from build123d import *

# Parameters (mm, degrees)
BOSS_EXTRUDE2_DEPTH     = 24
BOSS_EXTRUDE3_DEPTH     = 19
CUT_EXTRUDE1_DEPTH      = 1
BOSS_EXTRUDE4_DEPTH     = 50
SKETCH5_R               = 4
CUT_EXTRUDE2_DEPTH      = 55
SKETCH6_R               = 5
CUT_EXTRUDE3_DEPTH      = 25
CUT_EXTRUDE3_DEPTH_BACK = 25


with BuildPart() as part:
    # Sketch1 → Boss-Extrude2 (new body, symmetric)
    with BuildSketch(Plane.XY):
        Polygon((0, 0), (84, 0), (84, 19), (53, 19), (51.5, 16), (50, 19), (0, 19), align=None)
    extrude(amount=BOSS_EXTRUDE2_DEPTH, both=True)

    # Sketch2 → Boss-Extrude3 (add)
    with BuildSketch(Plane(origin=(0, 0, 0), x_dir=(1, 0, 0), z_dir=(0, 1, 0))):
        Polygon((84, 2), (89, 2), (100, 13.5), (100, 16.5), (89, 16.5), (89, 13.5), (84, 13.5), align=None)
    boss_extrude3 = extrude(amount=BOSS_EXTRUDE3_DEPTH)

    # Mirror1: Boss-Extrude3 across plane
    add(boss_extrude3.mirror(Plane.XY))

    # Sketch3 → Cut-Extrude1 (cut)
    with BuildSketch(Plane(origin=(0, 19, 0), x_dir=(1, 0, 0), z_dir=(0, 1, 0))):
        with BuildLine():
            Line((66, 12.5), (66, -12.5))
            ThreePointArc((66, -12.5), (63, -15.5), (60, -12.5))
            Line((60, -12.5), (60, 12.5))
            ThreePointArc((60, 12.5), (63, 15.5), (66, 12.5))
        make_face()
    extrude(amount=-CUT_EXTRUDE1_DEPTH, mode=Mode.SUBTRACT)

    # Sketch4 → Boss-Extrude4 (add)
    with BuildSketch(Plane(origin=(0, 0, 0), x_dir=(0, 0, -1), z_dir=(1, 0, 0))):
        Polygon((-18, 19), (-18, 32), (-24, 32), (-24, 38), (-13.5, 38), (-13.5, 43), (-16.5, 43), (-16.5, 54), (-13.5, 54), (-3.604820816, 41), (-3.604820816, 38), (0, 38), (0, 19), align=None)
    boss_extrude4 = extrude(amount=BOSS_EXTRUDE4_DEPTH)

    # Mirror2: Boss-Extrude4 across plane
    add(boss_extrude4.mirror(Plane.XY))

    # Sketch5 → Cut-Extrude2 (cut, through all)
    with BuildSketch(Plane(origin=(0, 0, 0), x_dir=(1, 0, 0), z_dir=(0, 1, 0))):
        with Locations((25, 0)):
            Circle(SKETCH5_R)
    extrude(amount=CUT_EXTRUDE2_DEPTH, mode=Mode.SUBTRACT)

    # Sketch6 → Cut-Extrude3 (cut, two sides)
    with BuildSketch(Plane.XY) as cut_extrude3_sk:
        with Locations((25, 25)):
            Circle(SKETCH6_R)
    extrude(amount=CUT_EXTRUDE3_DEPTH, mode=Mode.SUBTRACT)
    extrude(cut_extrude3_sk.sketch, amount=-CUT_EXTRUDE3_DEPTH_BACK, mode=Mode.SUBTRACT)


solid = part.part
For this review, take the finished solid that the model builds, in its own axes (mm). A direction names the side the tool comes from. Round coordinates to 2 decimals unless told otherwise and drop trailing zeros. Order: outer loops, then holes, each group sorted by start corner. A loop starts at its lowest first (then second) coordinate and runs counter-clockwise, first axis right, second up. Notation, with made-up numbers: M 27.5,89.25 L 71.5,89.25 A12 cw 71.5,111.25 Z; hole C 77.5,53 d1. An arc over 180 degrees is marked long. Use a Markdown table: item, result. Add a question column.
Item 1: Add section A-A, the plane y = 25. Give the boundary of the cut face in (x, z).
Item 2: To check wall thickness, follow line 1 along X through (y, z) = (21, 7); line 2 along X through (y, z) = (17, 0); line 3 along Z through (x, y) = (25, 31.5). State the ranges of each line that lie inside material, in increasing order.
Item 3: Add section B-B, the plane z = -19.5. Give the boundary of the cut face in (x, y).
Item 4: Add section D-D, the plane z = 9. Give the boundary of the cut face in (x, y), then the cut area to 3 significant figures.
Item 5: Mouldability with a two-part tool opening along Y and no side actions: class faces 1 (the flat face through (94.423, 9.367, -7.67)), 2 (the flat face through (25, 43, 15)) as released by +Y, released by -Y, zero draft, split by the parting line, or undercut.
Item 6: Insertion check: pin 1 (3.5 mm diameter, centred on x = 7.5, z = 0.5, fed in from +Y); pin 2 (5.5 mm diameter, centred on x = 87.5, y = 10, fed in from -Z); pin 3 (0.9 mm diameter, centred on x = 40, y = 39, fed in from +Z); pin 4 (4 mm diameter, centred on y = 43, z = 0.5, fed in from +X). Each pin has a flat end and moves straight along its axis. Give the tip position at first contact, or say it passes through.
Item 7: Tool access review of faces 3 (the flat face through (25, 40, -13.5)), 4 (the flat face through (25, 38, 19)), 5 (the flat face through (95, 9, -16.5)), 6 (the cylindrical face through (62.9, 18.5, -15.5)), 7 (the flat face through (94.423, 9.367, 7.67)): name each direction out of +Z, -Z, +X, -X, +Y, -Y from which nothing blocks a thin tool from reaching the whole face with its end or side.
Item 8: Add section C-C, the plane x = 63. Give the boundary of the cut face in (y, z), then the cut area to 3 significant figures.
Geometry results:
| question | item | result |
|---|---|---|
| 1 | outline | M 0,-18 L 20,-18 L 20,18 L 0,18 Z; M 30,-18 L 50,-18 L 50,18 L 30,18 Z |
| 2 | line 1 | x = 0 to 22, 28 to 50 |
| 2 | line 2 | x = 0 to 21, 29 to 51, 52 to 84 |
| 2 | line 3 | z = -18 to -4, 4 to 18 |
| 3 | outline | M 0,0 L 84,0 L 84,19 L 53,19 L 51.5,16 L 50,19 L 0,19 Z; M 0,32 L 50,32 L 50,38 L 0,38 Z |
| 4 | outline | M 0,0 L 95.7,0 L 95.7,19 L 66,19 L 66,18 L 60,18 L 60,19 L 53,19 L 51.5,16 L 50,19 L 50,48.09 L 0,48.09 Z; hole C 25,25 d10 |
| 4 | area | 3,180 mm² |
| 5 | face 1 | zero draft |
| 5 | face 2 | undercut |
| 6 | pin 1 | stops at y = 38 |
| 6 | pin 2 | stops at z = -16.5 |
| 6 | pin 3 | stops at z = 13.5 |
| 6 | pin 4 | passes through |
| 7 | face 3 | -Z, +X, -X |
| 7 | face 4 | +Z, +X, -X |
| 7 | face 5 | -Z, +X, +Y, -Y |
| 7 | face 6 | +Y |
| 7 | face 7 | +X, +Y, -Y |
| 8 | outline | M 0,-24 L 19,-24 L 19,-15.5 L 18,-15.5 L 18,15.5 L 19,15.5 L 19,24 L 0,24 Z |
| 8 | area | 881 mm² |
